```python
from build123d import *

# Parameters (mm, degrees)
SKETCH_1_W              = 140
SKETCH_1_H              = 148
SKETCH_1_W_2            = 80
SKETCH_1_H_2            = 46
EXTRUDE_1_DEPTH         = 4
HOLE_WIZARD_M4_1_D      = 4.5
HOLE_WIZARD_4_5_4_5_1_D = 4.5
SKETCH_9_W              = 65
SKETCH_9_H              = 140
EXTRUDE_3_DEPTH         = 4
HOLE_WIZARD_M2_1_D      = 2.4
CUT_EXTRUDE_1_DEPTH     = 255.921556562
HOLE_WIZARD_M3_1_D      = 3.4
FILLET_6_R              = 7.5
FILLET_8_R              = 3


with BuildPart() as part:
    # ｽｹｯﾁ1 → ﾎﾞｽ - 押し出し1 (new body)
    with BuildSketch(Plane(origin=(0, 0, 0), x_dir=(0, 1, 0), z_dir=(0, 0, 1))):
        with Locations((70, -74)):
            Rectangle(SKETCH_1_W, SKETCH_1_H)
        with Locations((70, -47)):
            Rectangle(SKETCH_1_W_2, SKETCH_1_H_2, mode=Mode.SUBTRACT)
        with Locations((70, -101)):
            Rectangle(SKETCH_1_W_2, SKETCH_1_H_2, mode=Mode.SUBTRACT)
    extrude(amount=EXTRUDE_1_DEPTH)

    # M4 すきま穴1 (through all)
    with Locations(Plane.XY.offset(4)):
        with Locations((7.5, 132.5), (140.5, 132.5), (7.5, 7.5), (140.5, 7.5)):
            Hole(HOLE_WIZARD_M4_1_D / 2)

    # Ø4.5 (4.5) 直径の穴1 (through all)
    with Locations(Plane.XY.offset(4)):
        with Locations((44, 117.5), (104, 117.5), (104, 22.5), (44, 22.5)):
            Hole(HOLE_WIZARD_4_5_4_5_1_D / 2)

    # ｽｹｯﾁ9 → ﾎﾞｽ - 押し出し3 (add)
    with BuildSketch(Plane.XY.offset(4)):
        with Locations((180.5, 70)):
            Rectangle(SKETCH_9_W, SKETCH_9_H)
    extrude(amount=-EXTRUDE_3_DEPTH)

    # M2 すきま穴1 (through all)
    with Locations(Plane.XY.offset(4)):
        with Locations((203, 10), (154, 68), (203, 68), (154, 10)):
            Hole(HOLE_WIZARD_M2_1_D / 2)

    # ｽｹｯﾁ13 → ｶｯﾄ - 押し出し1 (cut, through all)
    with BuildSketch(Plane.XY.offset(4)):
        Polygon((168.5, 125), (188.5, 125), (188.5, 103), (196, 103), (196, 15), (161, 15), (161, 103), (168.5, 103), align=None)
    extrude(amount=-CUT_EXTRUDE_1_DEPTH, mode=Mode.SUBTRACT)

    # M3 すきま穴1 (through all)
    with Locations(Plane.XY.offset(4)):
        with Locations((163.5, 114), (193.5, 114)):
            Hole(HOLE_WIZARD_M3_1_D / 2)

    # ﾌｨﾚｯﾄ6
    fillet_6_edges = [part.edges().sort_by_distance(p)[0] for p in [
        (168.5, 125, 2),
        (188.5, 125, 2),
        (196, 15, 2),
        (161, 15, 2),
        (24, 30, 2),
        (70, 30, 2),
        (70, 110, 2),
        (24, 110, 2),
        (124, 110, 2),
        (78, 110, 2),
        (78, 30, 2),
        (124, 30, 2),
        (0, 0, 2),
        (0, 140, 2),
        (213, 140, 2),
        (213, 0, 2),
    ]]
    fillet(fillet_6_edges, radius=FILLET_6_R)

    # ﾌｨﾚｯﾄ8
    fillet_8_edges = [part.edges().sort_by_distance(p)[0] for p in [
        (168.5, 103, 2),
        (188.5, 103, 2),
        (196, 103, 2),
        (161, 103, 2),
    ]]
    fillet(fillet_8_edges, radius=FILLET_8_R)


solid = part.part
```
Part model, mm, in its own coordinate system. Give positions to 0.01 mm unless a question says otherwise; leave off trailing zeros. Write each loop counter-clockwise with the first axis right and the second up, starting at its lowest first coordinate (ties: lowest second). Pieces come first, ordered by that corner, then holes. Notation, with made-up numbers: (61, -0.75) -> (120, -0.75) arc R21 ccw to (120, 19.25) -> close; hole circle Ø1 at (57.25, 78). An arc over 180 degrees is marked (long way). Put each result on its own line as item: value. Start each with the question number.
Item 1: Cut at D-D (z = 2.95). State how many separate pieces and enclosed holes the cut face has, then the cut area to 3 significant figures.
Item 2: Pin check, flat tips, straight feed: pin 1 Ø4 at (x, y) = (154, 68) entering from -Z; pin 2 Ø4 at (x, y) = (7.5, 7.5) entering from -Z. Stop position of each tip, or through.
Item 3: Wall check: L1, parallel to Y at x = 203, z = 2.05; L2, parallel to Y at x = 140.5, z = 2.4; L3, parallel to X at y = 68, z = 2.35. Give the ranges that are in metal, low to high. Write a range as [from, to].
Item 4: Cut at B-B (x = 104). List the corners of the cut face in (y, z).
Item 5: Cut at C-C (x = 80.5). List the corners of the cut face in (y, z), then the cut area to 3 significant figures.
Item 6: Cut at A-A (y = 45.5). List the corners of the cut face in (x, z).
Item 7: Pull direction X, two halves, no side cores. Call faces 1 (the face through (2.139, 137.745, 2.028)), 2 (the face through (105, 0, 2)), 3 (the face through (101.92, 21.64, 1.97)), 4 (the face through (210.745, 2.139, 1.972)): pulls with the +X half, pulls with the -X half, needs draft (parallel to the pull), parting line crosses it, or undercut.
Answer list:
1. separate pieces: 1
1. enclosed holes: 17
1. area: 18,900 mm2
2. pin 1: stops at z = 0
2. pin 2: passes through
3. L1: y = [0, 8.8], [11.2, 66.8], [69.2, 140]
3. L2: y = [0, 5.25], [9.75, 130.25], [134.75, 140]
3. L3: x = [0, 24], [70, 78], [124, 152.8], [155.2, 161], [196, 201.8], [204.2, 213]
4. outline: (0, 0) -> (20.25, 0) -> (20.25, 4) -> (0, 4) -> close; (24.75, 0) -> (30, 0) -> (30, 4) -> (24.75, 4) -> close; (110, 0) -> (115.25, 0) -> (115.25, 4) -> (110, 4) -> close; (119.75, 0) -> (140, 0) -> (140, 4) -> (119.75, 4) -> close
5. outline: (0, 0) -> (31.91, 0) -> (31.91, 4) -> (0, 4) -> close; (108.09, 0) -> (140, 0) -> (140, 4) -> (108.09, 4) -> close
5. area: 255 mm2
6. outline: (0, 0) -> (24, 0) -> (24, 4) -> (0, 4) -> close; (70, 0) -> (78, 0) -> (78, 4) -> (70, 4) -> close; (124, 0) -> (161, 0) -> (161, 4) -> (124, 4) -> close; (196, 0) -> (213, 0) -> (213, 4) -> (196, 4) -> close
7. face 1: pulls with the -X half
7. face 2: needs draft
7. face 3: undercut
7. face 4: pulls with the +X half
